```python
from build123d import *

# Parameters (mm, degrees)
MODEL_W             = 20
MODEL_H             = 5.35
MODEL_W_2           = 5.35
MODEL_H_2           = 10
MODEL_H_3           = 12
MODEL_W_3           = 11
MODEL_H_4           = 9
BOSS_EXTRUDE1_DEPTH = 5.35


with BuildPart() as part:
    # Model → Boss-Extrude1 (new body)
    with BuildSketch(Plane.XY):
        with BuildLine():
            Line((125, 304.11), (145, 304.11))
            Line((145, 304.11), (145, 265.61))
            Line((145, 265.61), (150.35, 265.61))
            Line((150.35, 265.61), (150.35, 218.943333333))
            Line((150.35, 218.943333333), (145, 218.943333333))
            Line((145, 218.943333333), (145, 180.443333333))
            Line((145, 180.443333333), (150.35, 180.443333333))
            Line((150.35, 180.443333333), (150.35, 133.776666667))
            Line((150.35, 133.776666667), (145, 133.776666667))
            Line((145, 133.776666667), (145, 95.276666667))
            Line((145, 95.276666667), (150.35, 95.276666667))
            Line((150.35, 95.276666667), (150.35, 48.61))
            Line((150.35, 48.61), (145, 48.61))
            Line((145, 48.61), (145, 10.11))
            Line((145, 10.11), (125, 10.11))
            Line((125, 10.11), (125, 15.46))
            Line((125, 15.46), (105, 15.46))
            Line((105, 15.46), (105, 0))
            Line((105, 0), (-105, 0))
            Line((-105, 0), (-105, 15.46))
            Line((-105, 15.46), (-125, 15.46))
            Line((-125, 15.46), (-125, 10.11))
            Line((-125, 10.11), (-145, 10.11))
            Line((-145, 10.11), (-145, 48.61))
            Line((-145, 48.61), (-150.35, 48.61))
            Line((-150.35, 48.61), (-150.35, 95.276666667))
            Line((-150.35, 95.276666667), (-145, 95.276666667))
            Line((-145, 95.276666667), (-145, 133.776666667))
            Line((-145, 133.776666667), (-150.35, 133.776666667))
            Line((-150.35, 133.776666667), (-150.35, 180.443333333))
            Line((-150.35, 180.443333333), (-145, 180.443333333))
            Line((-145, 180.443333333), (-145, 218.943333333))
            Line((-145, 218.943333333), (-150.35, 218.943333333))
            Line((-150.35, 218.943333333), (-150.35, 265.61))
            Line((-150.35, 265.61), (-145, 265.61))
            Line((-145, 265.61), (-145, 304.11))
            Line((-145, 304.11), (-125, 304.11))
            Line((-125, 304.11), (-125, 298.76))
            Line((-125, 298.76), (-105, 298.76))
            Line((-105, 298.76), (-105, 306.789491924))
            ThreePointArc((-105, 306.789491924), (-97.679491924, 314.11), (-95, 324.11))
            Line((-95, 324.11), (-95, 329.11))
            ThreePointArc((-95, 329.11), (-89.142135624, 343.252135624), (-75, 349.11))
            Line((-75, 349.11), (75, 349.11))
            ThreePointArc((75, 349.11), (89.142135624, 343.252135624), (95, 329.11))
            Line((95, 329.11), (95, 324.11))
            ThreePointArc((95, 324.11), (97.679491924, 314.11), (105, 306.789491924))
            Line((105, 306.789491924), (105, 298.76))
            Line((105, 298.76), (125, 298.76))
            Line((125, 298.76), (125, 304.11))
        make_face()
        with Locations((-115, 157.11)):
            Rectangle(MODEL_W, MODEL_H, mode=Mode.SUBTRACT)
        with Locations((-115, 228.19)):
            Rectangle(MODEL_W, MODEL_H, mode=Mode.SUBTRACT)
        with Locations((-115, 86.03)):
            Rectangle(MODEL_W, MODEL_H, mode=Mode.SUBTRACT)
        with Locations((-42.325, 192.65)):
            Rectangle(MODEL_W_2, MODEL_H_2, mode=Mode.SUBTRACT)
        with Locations((-42.325, 263.73)):
            Rectangle(MODEL_W_2, MODEL_H_2, mode=Mode.SUBTRACT)
        with Locations((-42.325, 121.57)):
            Rectangle(MODEL_W_2, MODEL_H_2, mode=Mode.SUBTRACT)
        with Locations((-42.325, 50.49)):
            Rectangle(MODEL_W_2, MODEL_H_2, mode=Mode.SUBTRACT)
        with Locations((-50, 304.275)):
            Rectangle(MODEL_W, MODEL_H, mode=Mode.SUBTRACT)
        with Locations((0, 8.675)):
            Rectangle(MODEL_W, MODEL_H, mode=Mode.SUBTRACT)
        with Locations((-82.325, 288.6)):
            Rectangle(MODEL_W_2, MODEL_H_3, mode=Mode.SUBTRACT)
        with Locations((-50, 8.675)):
            Rectangle(MODEL_W, MODEL_H, mode=Mode.SUBTRACT)
        with Locations((-82.325, 24.35)):
            Rectangle(MODEL_W_2, MODEL_H_3, mode=Mode.SUBTRACT)
        with Locations((0, 304.275)):
            Rectangle(MODEL_W, MODEL_H, mode=Mode.SUBTRACT)
        with Locations((-73.5, 336.625)):
            Rectangle(MODEL_W_3, MODEL_H, mode=Mode.SUBTRACT)
        with Locations((-44.825, 320.45)):
            Rectangle(MODEL_W_2, MODEL_H_4, mode=Mode.SUBTRACT)
        with Locations((-34.5, 336.625)):
            Rectangle(MODEL_W_3, MODEL_H, mode=Mode.SUBTRACT)
        with Locations((50, 304.275)):
            Rectangle(MODEL_W, MODEL_H, mode=Mode.SUBTRACT)
        with Locations((44.825, 320.45)):
            Rectangle(MODEL_W_2, MODEL_H_4, mode=Mode.SUBTRACT)
        with Locations((34.5, 336.625)):
            Rectangle(MODEL_W_3, MODEL_H, mode=Mode.SUBTRACT)
        with Locations((73.5, 336.625)):
            Rectangle(MODEL_W_3, MODEL_H, mode=Mode.SUBTRACT)
        with Locations((115, 86.03)):
            Rectangle(MODEL_W, MODEL_H, mode=Mode.SUBTRACT)
        with Locations((115, 157.11)):
            Rectangle(MODEL_W, MODEL_H, mode=Mode.SUBTRACT)
        with Locations((115, 228.19)):
            Rectangle(MODEL_W, MODEL_H, mode=Mode.SUBTRACT)
        with Locations((82.325, 288.6)):
            Rectangle(MODEL_W_2, MODEL_H_3, mode=Mode.SUBTRACT)
        with Locations((42.325, 263.73)):
            Rectangle(MODEL_W_2, MODEL_H_2, mode=Mode.SUBTRACT)
        with Locations((42.325, 192.65)):
            Rectangle(MODEL_W_2, MODEL_H_2, mode=Mode.SUBTRACT)
        with Locations((42.325, 121.57)):
            Rectangle(MODEL_W_2, MODEL_H_2, mode=Mode.SUBTRACT)
        with Locations((42.325, 50.49)):
            Rectangle(MODEL_W_2, MODEL_H_2, mode=Mode.SUBTRACT)
        with Locations((82.325, 24.35)):
            Rectangle(MODEL_W_2, MODEL_H_3, mode=Mode.SUBTRACT)
        with Locations((50, 8.675)):
            Rectangle(MODEL_W, MODEL_H, mode=Mode.SUBTRACT)
    extrude(amount=BOSS_EXTRUDE1_DEPTH)


solid = part.part
```
The listing builds one solid part. Answer for the finished solid, in the listing's coordinates (mm). Round coordinates to 2 decimals unless told otherwise and drop trailing zeros. Loops run counter-clockwise (first coordinate to the right, second up) from the corner with the lowest first, then second, coordinate; pieces in that order, holes last. Notation, with made-up numbers: (38.5, 9) -> (95.5, 9) arc R13 ccw to (95.5, 19) -> close; hole circle Ø10 at (38.25, 16). An arc over 180 degrees is marked (long way). Use one line per item in the form item = value.
1. Flat-ended cylindrical pins translate along their axes: pin 1 Ø3 at (y, z) = (103.5, 0.5) entering from -X; pin 2 Ø2.5 at (x, z) = (149, 4) entering from -Y; pin 3 Ø1.6 at (x, z) = (-112.5, 2) entering from +Y. Find the tip coordinate at first contact, or state that the pin passes through.
Answer key:
pin_1 = -145
pin_2 = 48.61
pin_3 = 298.76
2. The part is cut by section B-B on y = 203. Determine the outline of the cut face in (x, z), and give its area (3 significant figures).
Answer key:
outline = (-145, 0) -> (145, 0) -> (145, 5.35) -> (-145, 5.35) -> close
area = 1,550 mm²
3. Find the intervals of material crossed by probe 1 along X at (y, z) = (194.5, 1.1); probe 2 along Y at (x, z) = (58.5, 1.3); probe 3 along X at (y, z) = (306, 2.05), in increasing order. Write a range as [from, to].
Answer key:
probe_1 = [-145, -45], [-39.65, 39.65], [45, 145]
probe_2 = [0, 6], [11.35, 301.6], [306.95, 349.11]
probe_3 = [-105, -60], [-40, -10], [10, 40], [60, 105]
4. The part is cut by section A-A on z = 3.5. Give the number of separate pieces and of enclosed holes in the cut face, and give its area (3 significant figures).
Answer key:
separate_pieces = 1
enclosed_holes = 30
area = 94,700 mm²
